Design review of the part shown in the three views and the two pictorial views. Dimensions are in mm from the part's minimum x, y and z. Coordinates: 2 decimals unless noted, no trailing zeros. Loops run counter-clockwise (first coordinate to the right, second up) from the corner with the lowest first, then second, coordinate; pieces in that order, holes last. Notation, with made-up numbers: M -12,-18.5 L -1,-18.5 A26 ccw -1,-2.5 Z; hole C 54.25,81 d5. An arc over 180 degrees is marked long. Put each result on its own line as item: value. Start each with the question number.
(1) For probe 1 along Y at (x, z) = (72.5, 26.5); probe 2 along Y at (x, z) = (125, 30) (1 decimal); probe 3 along Z at (x, y) = (80, 13.5), list the stretches that pass through material, from the lowest coordinate up. Write a range as [from, to].
(2) Take a section at A-A, the plane x = 72.5. Give the boundary of the cut face in (y, z), then the cut area to 3 significant figures.
(3) Take a section at C-C, the plane y = 42. Give the boundary of the cut face in (x, z), then the cut area to 3 significant figures.
(4) The part is to be moulded in two halves that separate along Y. For the marked faces 1 and 2, say which applies: +Y half, -Y half, draft (parallel to the pull), parting line (faces both ways), or undercut.
(5) Take a section at B-B, the plane y = 72.5. Give the boundary of the cut face in (x, z), then the cut area to 3 significant figures.
(6) Take a section at D-D, the plane z = 25. Give the boundary of the cut face in (x, y), then the cut area to 3 significant figures.
(7) Clearance check with flat-ended pins moving along their axes: pin 1 (1 mm diameter, centred on x = 69, z = 15.5, fed in from +Y); pin 2 (3 mm diameter, centred on x = 122, z = 22, fed in from -Y) (1 decimal); pin 3 (1 mm diameter, centred on y = 62.5, z = 28, fed in from -X) (1 decimal). State where each tip first meets the part, or that it passes through.
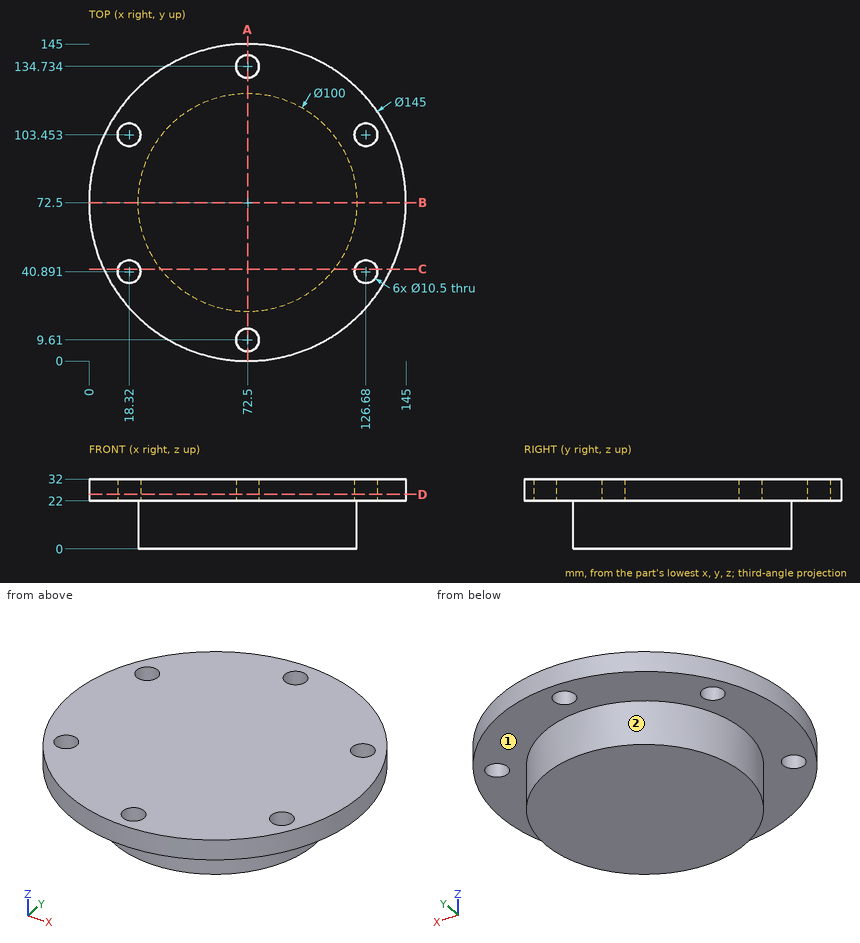
Computed values:
1. probe 1: y = [0, 4.36], [14.86, 129.48], [139.98, 145]
1. probe 2: y = [22.5, 35.9], [45.9, 98.5], [108.4, 122.5]
1. probe 3: z = [22, 32]
2. outline: M 0,22 L 4.36,22 L 4.36,32 L 0,32 Z; M 14.86,22 L 22.5,22 L 22.5,0 L 122.5,0 L 122.5,22 L 129.48,22 L 129.48,32 L 14.86,32 Z; M 139.98,22 L 145,22 L 145,32 L 139.98,32 Z
2. area: 3,440 mm^2
3. outline: M 6.73,22 L 13.19,22 L 13.19,32 L 6.73,32 Z; M 23.45,22 L 32.88,22 L 32.88,0 L 112.12,0 L 112.12,22 L 121.55,22 L 121.55,32 L 23.45,32 Z; M 131.81,22 L 138.27,22 L 138.27,32 L 131.81,32 Z
3. area: 2,850 mm^2
4. face 1: draft
4. face 2: parting line
5. outline: M 0,22 L 22.5,22 L 22.5,0 L 122.5,0 L 122.5,22 L 145,22 L 145,32 L 0,32 Z
5. area: 3,650 mm^2
6. outline: C 72.5,72.5 d145; hole C 18.32,40.89 d10.5; hole C 18.32,103.45 d10.5; hole C 72.5,9.61 d10.5; hole C 72.5,134.73 d10.5; hole C 126.68,40.89 d10.5; hole C 126.68,103.45 d10.5
6. area: 16,000 mm^2
7. pin 1: stops at y = 122.41
7. pin 2: stops at y = 18.2
7. pin 3: stops at x = 0.6
